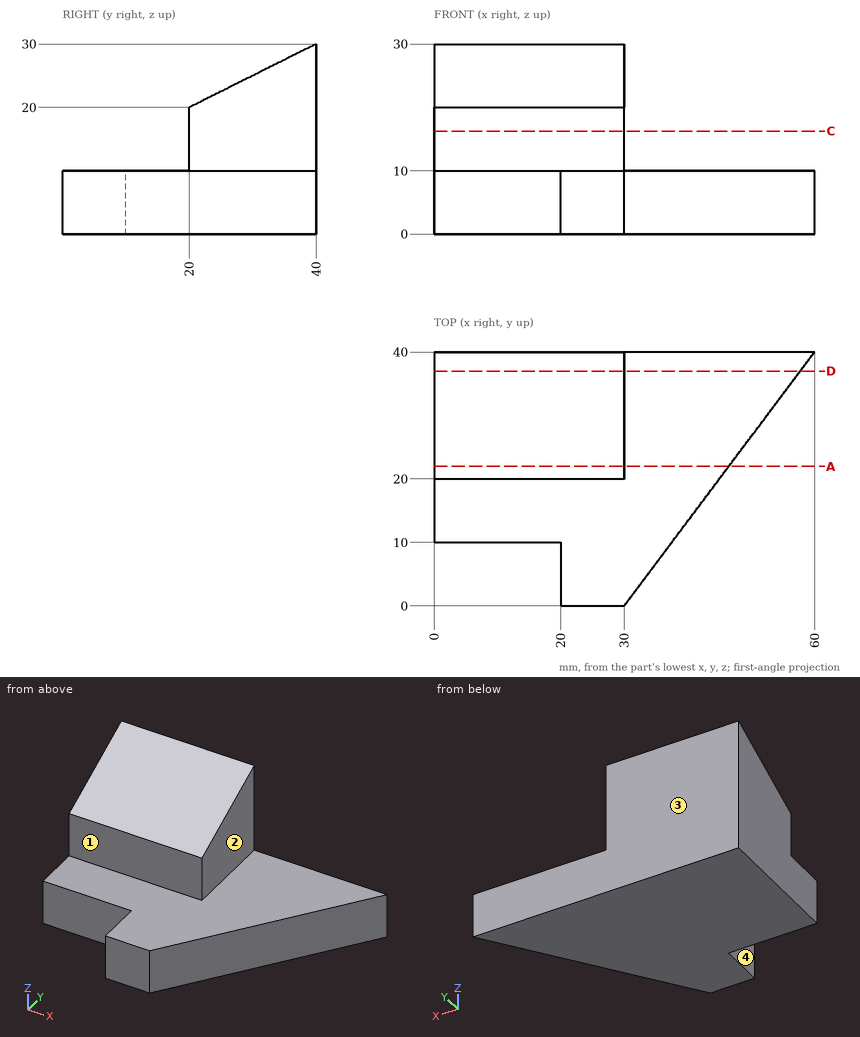
Study the drawing (mm; zero at the part's minimum x, y, z) and answer. A direction names the side the tool comes from. Give positions to 0.01 mm unless a question says otherwise; leave off trailing zeros. Write each loop counter-clockwise with the first axis right and the second up, starting at its lowest first coordinate (ties: lowest second). Pieces come first, ordered by that corner, then holes.
(1) Flat-ended cylindrical pins translate along their axes: pin 1 Ø2 at (x, z) = (18.5, 17) entering from -Y; pin 2 Ø10 at (y, z) = (25.5, 18) entering from +X; pin 3 Ø1.5 at (x, y) = (25.5, 4) entering from +Z. Find the tip coordinate at first contact, or state that the pin passes through.
Final values:
pin 1: stops at y = 20
pin 2: stops at x = 30
pin 3: stops at z = 10
(2) The part is cut by section D-D on y = 37. Write down the section's boundary in (x, z).
Final values:
outline: (0, 0) - (57.75, 0) - (57.75, 10) - (30, 10) - (30, 28.5) - (0, 28.5) - close
(3) The part is cut by section C-C on z = 16.25. Write down the section's boundary in (x, y), plus the area to 3 significant figures.
Final values:
outline: (0, 20) - (30, 20) - (30, 40) - (0, 40) - close
area: 600 mm2
(4) Which of the six approach directions +Z, -Z, +X, -X, +Y, -Y give full straight-line access (tool end or side, diameter ignored) to the marked faces 1, 2, 3 and 4?
Final values:
face 1: +Z, +X, -X, -Y
face 2: +Z, +X, +Y, -Y
face 3: +Z, -Z, +X, -X, +Y
face 4: +Z, -Z, -X, -Y
(5) Straight lines are drawn through the part: line 1 (X direction, y = 27.5, z = 13.5); line 2 (Z direction, x = 48, y = 30); line 3 (Y direction, x = 24.5, z = 19.5). For each, find the intervals that lie inside material, in ascending order.
Final values:
line 1: x = 0 to 30
line 2: z = 0 to 10
line 3: y = 20 to 40
(6) The part is cut by section A-A on y = 22. Write down the section's boundary in (x, z).
Final values:
outline: (0, 0) - (46.5, 0) - (46.5, 10) - (30, 10) - (30, 21) - (0, 21) - close
